Source: CAD feature listing. Evaluate the final solid. Frame: model axes, mm. A direction names the side the tool comes from. Round coordinates to 2 decimals unless told otherwise and drop trailing zeros. Loops run counter-clockwise (first coordinate to the right, second up) from the corner with the lowest first, then second, coordinate; pieces in that order, holes last. Notation, with made-up numbers: (45.5, 5.25) -> (51.5, 5.25) arc R13 ccw to (51.5, 11.25) -> close; hole circle Ø1 at (73.5, 65). An arc over 180 degrees is marked (long way). Put each result on its own line as item: value. Start each with the question number.
1. Set-up query: faces 4 (the flat face through (17, 20, 0)), 5 (the flat face through (63.5, 40, 2)), 6 (the flat face through (55, 0, -27)), 7 (the flat face through (55.88, -2, -40)). Return all of +Z, -Z, +X, -X, +Y, -Y with unobstructed straight access to the full face (end or side cutting, diameter ignored); none if empty.
2. Cut plane A-A (z = -40). Return the cut outline in (x, y) (1 decimal), then the cut area to 3 significant figures.
3. Cut plane D-D (y = 11). Return the cut outline in (x, z) (1 decimal), then the cut area to 3 significant figures.
4. Contact query for flat-ended pins moving along their axis: pin 1 (24 mm diameter, centred on y = 35, z = -14, fed in from +X); pin 2 (5 mm diameter, centred on x = 49.5, y = 31.5, fed in from -Z); pin 3 (1 mm diameter, centred on x = 43, z = -6, fed in from +Y). Output: stop coordinate, or through.
5. Cut plane C-C (x = 16.51). Return the cut outline in (y, z) (3 decimals).
6. Draft query along X for faces 1 (the cylindrical face through (59.606, -1.565, -24.766)), 2 (the flat face through (76.2, 10, 1)), 3 (the cylindrical face through (1.91, 48.99, 1.61)). Return one class per face: pulls with the +X half, pulls with the -X half, needs draft (parallel to the pull), parting line crosses it, or undercut.
7. Cut plane B-B (y = 40.5). Return the cut outline in (x, z) (1 decimal).
8. Material intervals for L1, parallel to Z at x = 26.5, y = 25 (3 decimals); L2, parallel to X at y = 16.5, z = -30.5; L3, parallel to Y at x = 49, z = -15 (3 decimals), sorted ascending.
```python
from build123d import *

# Parameters (mm, degrees)
EXTRUDE_THIN1_DEPTH = 76.2
FILLET1_R           = 6.35
BOSS_EXTRUDE1_REACH = 88.253
SKETCH2_W           = 3.175
SKETCH2_H           = 71.842048968
CUT_EXTRUDE1_DEPTH  = 105.726882891
CUT_EXTRUDE2_DEPTH  = 105.726882891
FILLET2_R           = 1.524


with BuildPart() as part:
    # Sketch1 → Extrude-Thin1 (new body)
    with BuildSketch(Plane(origin=(0, 0, 0), x_dir=(0, 0, -1), z_dir=(1, 0, 0))):
        Polygon((50.8, 0), (0, 0), (0, 50.8), (-3.175, 50.8), (-3.175, -3.175), (50.8, -3.175), align=None)
    extrude(amount=EXTRUDE_THIN1_DEPTH)

    # Fillet1
    fillet1_edges = [part.edges().sort_by_distance(p)[0] for p in [
        (76.2, -1.5875, -50.8),
        (0, -1.5875, -50.8),
        (0, 50.8, 1.5875),
        (76.2, 50.8, 1.5875),
    ]]
    fillet(fillet1_edges, radius=FILLET1_R)

    # Sketch2 → Boss-Extrude1 (add, up to next)
    with BuildSketch(Plane(origin=(0, 25.4, -25.4), x_dir=(1, 0, 0), z_dir=(0, -0.7071067811865477, 0.7071067811865475)), mode=Mode.PRIVATE) as boss_extrude1_sk1:
        with Locations((38.1, 0)):
            Rectangle(SKETCH2_W, SKETCH2_H)
    boss_extrude1_tool1 = extrude(boss_extrude1_sk1.sketch, amount=BOSS_EXTRUDE1_REACH, mode=Mode.PRIVATE) - part.part
    add(boss_extrude1_tool1.solids().sort_by_distance((38.1, 25.4, -25.4))[0])

    # Sketch3 → Cut-Extrude1 (cut, through all)
    with BuildSketch(Plane.XY):
        with BuildLine():
            Line((12.7, 28.575), (12.7, 73.025))
            ThreePointArc((12.7, 73.025), (16.51, 76.835), (20.32, 73.025))
            Line((20.32, 73.025), (20.32, 28.575))
            ThreePointArc((20.32, 28.575), (16.51, 24.765), (12.7, 28.575))
        make_face()
        with BuildLine():
            Line((63.5, 28.575), (63.5, 73.025))
            ThreePointArc((63.5, 73.025), (59.69, 76.835), (55.88, 73.025))
            Line((55.88, 73.025), (55.88, 28.575))
            ThreePointArc((55.88, 28.575), (59.69, 24.765), (63.5, 28.575))
        make_face()
    extrude(amount=CUT_EXTRUDE1_DEPTH, mode=Mode.SUBTRACT)

    # Sketch4 → Cut-Extrude2 (cut, through all)
    with BuildSketch(Plane(origin=(0, 0, 0), x_dir=(1, 0, 0), z_dir=(0, 1, 0))):
        with BuildLine():
            Line((20.32, 73.025), (20.32, 28.575))
            ThreePointArc((20.32, 28.575), (16.51, 24.765), (12.7, 28.575))
            Line((12.7, 28.575), (12.7, 73.025))
            ThreePointArc((12.7, 73.025), (16.51, 76.835), (20.32, 73.025))
        make_face()
        with BuildLine():
            Line((55.88, 73.025), (55.88, 28.575))
            ThreePointArc((55.88, 28.575), (59.69, 24.765), (63.5, 28.575))
            Line((63.5, 28.575), (63.5, 73.025))
            ThreePointArc((63.5, 73.025), (59.69, 76.835), (55.88, 73.025))
        make_face()
    extrude(amount=-CUT_EXTRUDE2_DEPTH, mode=Mode.SUBTRACT)

    # Fillet2
    fillet2_edges = [part.edges().sort_by_distance(p)[0] for p in [
        (18.25625, 0, 0),
        (39.6875, 25.4, 0),
        (36.5125, 25.4, 0),
        (39.6875, 0, -25.4),
        (36.5125, 0, -25.4),
        (57.94375, 0, 0),
    ]]
    fillet(fillet2_edges, radius=FILLET2_R)


solid = part.part
```
Solution:
1. face 4: -Z, -X, +Y
1. face 5: +Z, -Z, +Y
1. face 6: -Z, +X, +Y
1. face 7: -Z, +Y, -Y
2. outline: (0, -3.2) -> (12.7, -3.2) -> (12.7, 0) -> (0, 0) -> close; (20.3, -3.2) -> (55.9, -3.2) -> (55.9, 0) -> (41.2, 0) arc R1.5 cw to (39.7, 1.5) -> (39.7, 10.8) -> (36.5, 10.8) -> (36.5, 1.5) arc R1.5 cw to (35, 0) -> (20.3, 0) -> close; (63.5, -3.2) -> (76.2, -3.2) -> (76.2, 0) -> (63.5, 0) -> close
2. area: 229 mm^2
3. outline: (0, 0) -> (35, 0) arc R1.5 cw to (36.5, -1.5) -> (36.5, -39.8) -> (39.7, -39.8) -> (39.7, -1.5) arc R1.5 cw to (41.2, 0) -> (76.2, 0) -> (76.2, 3.2) -> (0, 3.2) -> close
3. area: 369 mm^2
4. pin 1: stops at x = 39.69
4. pin 2: stops at z = 0
4. pin 3: stops at y = 0
5. outline: (-3.175, -24.765) -> (0, -24.765) -> (0, -1.524) arc R1.524 cw to (1.524, 0) -> (24.765, 0) -> (24.765, 3.175) -> (-3.175, 3.175) -> close
6. face 1: undercut
6. face 2: pulls with the +X half
6. face 3: pulls with the -X half
7. outline: (0, 0) -> (12.7, 0) -> (12.7, 3.2) -> (0, 3.2) -> close; (20.3, 0) -> (35, 0) arc R1.5 cw to (36.5, -1.5) -> (36.5, -10.3) -> (39.7, -10.3) -> (39.7, -1.5) arc R1.5 cw to (41.2, 0) -> (55.9, 0) -> (55.9, 3.2) -> (20.3, 3.2) -> close; (63.5, 0) -> (76.2, 0) -> (76.2, 3.2) -> (63.5, 3.2) -> close
8. L1: z = 0 to 3.175
8. L2: x = 36.51 to 39.69
8. L3: y = -3.175 to 0
